```python
from build123d import *

# Parameters (mm, degrees)
F0_W     = 231.14
F0_H     = 226.06
F1_DEPTH = 241.3
F2_W     = 113.03
F2_H     = 76.2
F2_W_2   = 39.37
F2_W_3   = 150.0068409762
F2_H_2   = 43.18
F2_W_4   = 191.77
F3_DEPTH = 226.061
F6_DEPTH = 241.301
F4_W     = 102.87
F4_H     = 43.18
F4_W_2   = 39.37
F7_DEPTH = 114.046


# Not quite as in the source:
# - a feature names something its author has since deleted; it is built from what else it names


with BuildPart() as f1:
    # F0 (on Top) → F1 (new body)
    with BuildSketch(Plane.XY):
        with BuildLine():
            Line((-173.0334059873, -173.7446556775), (-173.0334059873, 52.3153443225))
            ThreePointArc((-173.0334059873, 52.3153443225), (-286.0634059873, -60.7146556775), (-173.0334059873, -173.7446556775))
        make_face()
        with Locations((-57.4634059873, -60.7146556775)):
            Rectangle(F0_W, F0_H)
        with BuildLine():
            ThreePointArc((58.1065940127, -173.7446556775), (171.1365940127, -60.7146556775), (58.1065940127, 52.3153443225))
            Line((58.1065940127, 52.3153443225), (58.1065940127, -173.7446556775))
        make_face()
    extrude(amount=F1_DEPTH)

    # F2 (on face) → F3 (cut, through all)
    with BuildSketch(Plane.XZ.offset(173.7446556775)):
        Polygon((18.7365940127, 241.3), (-82.8634059873, 241.3), (18.7365940127, 165.1), align=None)
        with Locations((114.6215940127, 203.2)):
            Rectangle(F2_W, F2_H)
        with Locations((38.4215940127, 203.2)):
            Rectangle(F2_W_2, F2_H)
        with Locations((-248.0368264754, 21.59)):
            Rectangle(F2_W_3, F2_H_2)
        with Locations((-77.1484059873, 21.59)):
            Rectangle(F2_W_4, F2_H_2)
    extrude(amount=-F3_DEPTH, mode=Mode.SUBTRACT)

    # F5 (on face) → F6 (cut, through all)
    with BuildSketch(Plane(origin=(0, 0, 0), x_dir=(1, 0, 0), z_dir=(0, 0, -1))):
        with BuildLine():
            ThreePointArc((-173.0334059873, 170.5696556775), (-282.8884059873, 60.7146556775), (-173.0334059873, -49.1403443225))
            Line((-173.0334059873, -49.1403443225), (3.4965941633, -49.1403443225))
            Line((3.4965941633, -49.1403443225), (18.7365940127, -49.1403443225))
            Line((18.7365940127, -49.1403443225), (18.7365940127, 170.5696556775))
            Line((18.7365940127, 170.5696556775), (3.4965941633, 170.5696556775))
            Line((3.4965941633, 170.5696556775), (-173.0334059873, 170.5696556775))
        make_face()
        with BuildLine():
            Line((18.7365940127, 170.5696556775), (18.7365940127, -49.1403443225))
            Line((18.7365940127, -49.1403443225), (21.9115940127, -49.1403443225))
            Line((21.9115940127, -49.1403443225), (58.1065940127, -49.1403443225))
            ThreePointArc((58.1065940127, -49.1403443225), (167.9615940127, 60.7146556775), (58.1065940127, 170.5696556775))
            Line((58.1065940127, 170.5696556775), (21.9115940127, 170.5696556775))
            Line((21.9115940127, 170.5696556775), (18.7365940127, 170.5696556775))
        make_face()
    extrude(amount=-F6_DEPTH, mode=Mode.SUBTRACT)

    # F4 (on face) → F7 (cut)
    with BuildSketch(Plane(origin=(0, 52.3153443225, 0), x_dir=(-1, 0, 0), z_dir=(0, 1, 0))):
        with Locations((-109.5415940127, 21.59)):
            Rectangle(F4_W, F4_H)
        with Locations((-38.4215940127, 21.59)):
            Rectangle(F4_W_2, F4_H)
    extrude(amount=-F7_DEPTH, mode=Mode.SUBTRACT)


solid = f1.part
```
Check sheet for the modelled part. Datum: model origin and axes. Units: mm. A direction names the side the tool comes from. Round coordinates to 2 decimals unless told otherwise and drop trailing zeros. Write each loop counter-clockwise with the first axis right and the second up, starting at its lowest first coordinate (ties: lowest second). Pieces come first, ordered by that corner, then holes. Notation, with made-up numbers: (11.5, 23) -> (54.5, 23) arc R31 ccw to (54.5, 52) -> close; hole circle Ø5 at (22.25, -39.5). An arc over 180 degrees is marked (long way). Put each result on its own line as item: value.
(1) Sectioned sample at C-C (z = 72). Enter the section's corners in (x, y) (3 decimals), plus the area to 3 significant figures.
Values found:
outline: (-173.033, -173.745) -> (58.107, -173.745) arc R113.03 ccw to (58.107, 52.315) -> (-173.033, 52.315) arc R113.03 ccw to start; hole (-173.033, -170.57) -> (58.107, -170.57) arc R109.855 ccw to (58.107, 49.14) -> (-173.033, 49.14) arc R109.855 ccw to start
area: 3,690 mm^2
(2) Sectioned sample at B-B (y = -70). Enter the section's corners in (x, z), plus the area to 3 significant figures.
Values found:
outline: (-285.68, 43.18) -> (-282.5, 43.18) -> (-282.5, 241.3) -> (-285.68, 241.3) -> close; (167.57, 0) -> (170.75, 0) -> (170.75, 165.1) -> (167.57, 165.1) -> close
area: 1,160 mm^2
(3) Go/stop test with flat-tipped pins: pin 1 Ø1.6 at (y, z) = (-172.5, 23) entering from -X; pin 2 Ø2 at (y, z) = (-51.5, 191) entering from +X; pin 3 Ø12 at (x, z) = (-184.5, 94.5) entering from -Y. Record where each tip stops, or that it passes through.
Values found:
pin 1: stops at x = 18.74
pin 2: stops at x = -282.41
pin 3: stops at y = -173.61
(4) Sectioned sample at D-D (z = 25.5). Enter the section's corners in (x, y) (3 decimals).
Values found:
outline: (18.737, -173.745) -> (58.107, -173.745) arc R113.03 ccw to (160.977, -13.879) -> (160.977, -22.167) arc R109.855 cw to (58.107, -170.57) -> (18.737, -170.57) -> close
(5) Tool access check on faces 1 (the face through (-59, 52.315, 119)), 2 (the face through (167.935, -58.299, 81.394)), 3 (the face through (168, -70, 165.1)). Record the directions out of +Z, -Z, +X, -X, +Y, -Y that give a thin tool (end or side, any length) a straight path to the whole face; none if there is none.
Values found:
face 1: +Z, -Z, +X, -X, +Y
face 2: +Z, -Z
face 3: +Z, +X, +Y, -Y
(6) Mould release check, pull along Y, two halves, no side actions. Record for faces 4 (the face through (-282.86, -63.13, 140.85)), 5 (the face through (171.11, -63.2, 81.39)), 6 (the face through (-32.77, 50.71, 203.73)): released by +Y, released by -Y, zero draft, split by the parting line, or undercut.
Values found:
face 4: undercut
face 5: split by the parting line
face 6: zero draft
(7) Sectioned sample at A-A (x = 28). Enter the section's corners in (y, z).
Values found:
outline: (-173.74, 0) -> (-170.57, 0) -> (-170.57, 165.1) -> (-173.74, 165.1) -> close; (49.14, 43.18) -> (52.32, 43.18) -> (52.32, 165.1) -> (49.14, 165.1) -> close
(8) Material ranges on line 1 (Y direction, x = -104, z = 116); line 2 (X direction, y = -56.5, z = 54.5); line 3 (X direction, y = -65.5, z = 115), recorded low to high.
Values found:
line 1: y = -173.74 to -170.57, 49.14 to 52.32
line 2: x = -285.98 to -282.81, 167.88 to 171.06
line 3: x = -285.96 to -282.78, 167.86 to 171.04
